Autodesk Inventor part; units mm, degrees
ref_plane "YZ Plane" through (0, 0, 0) normal (1, 0, 0) x (0, 1, 0)
ref_plane "XZ Plane" through (0, 0, 0) normal (0, 1, 0) x (-1, 0, 0)
ref_plane "XY Plane" through (0, 0, 0) normal (0, 0, 1) x (1, 0, 0)
sketch "Sketch1" plane through (0, 0, 0) normal (0, 1, 0) x (-1, 0, 0)
  line L0 (0, 0) -> (50, 0)
  line L1 (50, 0) -> (50, -50)
  line L2 (50, -50) -> (0, -50)
  line L3 (0, -50) -> (0, 0)
  dimension "d0" = 50
  dimension "d1" = 50
extrude "Extrusion1" add sketch "Sketch1" along normal blind 10
sketch "Sketch2" plane through (0, 10, 0) normal (0, 1, 0) x (1, 0, 0)
  line L0 (-31, 0) -> (-26, 0)
  line L1 (-26, 0) -> (-26, 50)
  line L2 (-26, 50) -> (-31, 50)
  line L3 (-31, 50) -> (-31, 0)
  line L4 (-50, 0) -> (0, 0)
  line L5 (0, 50) -> (-50, 50)
  line L6 (-19, 0) -> (-24, 0)
  line L7 (-24, 0) -> (-24, 50)
  line L8 (-24, 50) -> (-19, 50)
  line L9 (-19, 50) -> (-19, 0)
  line L10 (0, 0) -> (0, 50)
  dimension "d7" = 5
  dimension "d8" = 5
  dimension "d9" = 2
  dimension "d10" = 19
extrude "Extrusion2" add sketch "Sketch2" along normal blind 10 contours L3 L2 L1 L0 | L7 L5 L9 L4
fillet "Fillet1" radius 10 2 edges at (-19, 10, -25) (-31, 10, -25)
fillet "Fillet2" radius 10 6 edges at (0, 10, -25) (0, 5, -50) (-50, 5, -50) (-50, 5, 0) (0, 5, 0) (-50, 10, -25)
properties part number "CalibrationWallMounts"
Geometry check sheet. Reference: the model listing, model coordinates, mm. A direction names the side the tool comes from. Round coordinates to 2 decimals unless told otherwise and drop trailing zeros. Write each loop counter-clockwise with the first axis right and the second up, starting at its lowest first coordinate (ties: lowest second). Pieces come first, ordered by that corner, then holes. Notation, with made-up numbers: (58.5, 20) -> (109.5, 20) arc R20 cw to (109.5, 44) -> close; hole circle Ø2 at (57, -19). An arc over 180 degrees is marked (long way). Put each result on its own line as item: value.
1) Release check for a two-part mould opening along X. For faces 3 (the face through (-24, 15, -25)), 4 (the face through (-4, 4, -2)), 5 (the face through (-25, 0, -25)) record: pulls with the +X half, pulls with the -X half, needs draft (parallel to the pull), parting line crosses it, or undercut.
Recorded:
face 3: undercut
face 4: pulls with the +X half
face 5: needs draft
2) Thickness scan on probe 1 along Y at (x, z) = (-24.5, -16.5); probe 2 along X at (y, z) = (17.25, -20.5); probe 3 along X at (y, z) = (17.5, -44.5). Record the ranges inside material, lowest first. Write a range as from..to.
Recorded:
probe 1: y = 0..10
probe 2: x = -31.39..-26, -24..-18.61
probe 3: x = -31.32..-26, -24..-18.68
3) Cross-section at A-A, the plane y = 13.75. Enter the section's corners in (x, z).
Recorded:
outline: (-33.19, -50) -> (-26, -50) -> (-26, 0) -> (-33.19, 0) -> close; (-24, -50) -> (-16.81, -50) -> (-16.81, 0) -> (-24, 0) -> close
4) Access from +Z, -Z, +X, -X, +Y, -Y to the whole of each face (thin tool, end or side, straight path). Record for faces 1 (the face through (-25, 10, -25)), 2 (the face through (-16.319, 13.185, -24.65)).
Recorded:
face 1: +Z, -Z, +Y
face 2: +Z, -Z, +X, +Y
5) Cross-section at D-D, the plane x = -7.5. Enter the section's corners in (y, z), plus the area to 3 significant figures.
Recorded:
outline: (0, -49.68) -> (9.71, -49.68) -> (9.71, -0.32) -> (0, -0.32) -> close
area: 479 mm2
6) Cross-section at C-C, the plane y = 2.25. Enter the section's corners in (x, z).
Recorded:
outline: (-49.75, -42.22) arc R10 ccw to (-40, -50) -> (-10, -50) arc R10 ccw to (-0.25, -42.22) -> (-0.25, -7.78) arc R10 ccw to (-10, 0) -> (-40, 0) arc R10 ccw to (-49.75, -7.78) -> close
7) Depth check by flat-ended pin: P1, Ø8, axis at x = -10, z = -21.5, coming from the +Y side; P2, Ø8, axis at y = 16.5, z = -43, coming from the +X side; P3, Ø1.5, axis at y = 8.5, z = -33.5, coming from the -X side. Enter the tip coordinate at first touch or a pass-through.
Recorded:
P1: stops at y = 11.34
P2: stops at x = -15.61
P3: stops at x = -46.35
